Check sheet for the modelled part. Datum: model origin and axes. Units: mm. Face numbers are marked on the shaded views. A direction names the side the tool comes from. Give positions to 0.01 mm unless a question says otherwise; leave off trailing zeros. Order: outer loops, then holes, each group sorted by start corner. A loop starts at its lowest first (then second) coordinate and runs counter-clockwise, first axis right, second up.
Item 1: Sectioned sample at A-A on z = 10. Record the boundary of the cut face in (x, y).
Item 2: Sectioned sample at C-C on y = 26.5. Record the boundary of the cut face in (x, z).
Item 3: Material ranges on line 1 along X through (y, z) = (-8.7, 10); line 2 along X through (y, z) = (16.5, 1.5); line 3 along Z through (x, y) = (5.25, -9.1), recorded low to high.
Item 4: Release check for a two-part mould opening along X. For the marked faces 6, 7 and 8 record: released by +X, released by -X, zero draft, split by the parting line, or undercut.
Item 5: Sectioned sample at B-B on x = -29.75. Record the boundary of the cut face in (y, z), and give its area (3 significant figures).
Item 6: Sectioned sample at D-D on z = 5.75. Record the boundary of the cut face in (x, y).
Item 7: Access from +Z, -Z, +X, -X, +Y, -Y to the whole of each face (thin tool, end or side, straight path). Record for the marked faces 1, 2, 3, 4 and 5.
Item 8: Gauge pin test, flat ends, axial feed: P1, Ø1.8, axis at x = 5.25, z = 10, coming from the +Y side; P2, Ø12, axis at y = 8.5, z = 5.5, coming from the -X side; P3, Ø11.5, axis at x = 5, z = 9.5, coming from the +Y side; P4, Ø5, axis at x = -16, z = 5, coming from the -Y side. Record the tip position at first contact, or that the pin passes through.
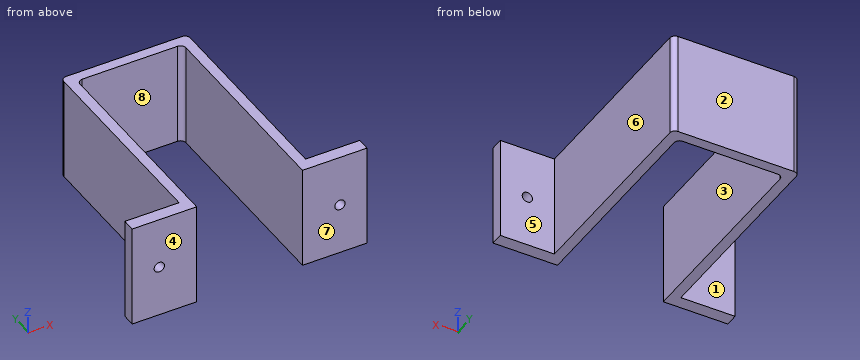
from build123d import *

# Parameters (mm, degrees)
BOSS_EXTRUDE1_DEPTH = 20
FILLET1_R           = 1
SKETCH2_R           = 1
CUT_EXTRUDE1_DEPTH  = 20


with BuildPart() as part:
    # Sketch1 → Boss-Extrude1 (new body)
    with BuildSketch(Plane.XY):
        Polygon((-22.5, -10.265235457), (-22.5, 30.234764543), (-2, 30.234764543), (-2, -10.265235457), (0, -10.265235457), (10.5, -10.265235457), (10.5, -7.797091413), (0, -7.797091413), (0, 32.234764543), (-24.5, 32.234764543), (-24.5, -7.797091413), (-35, -7.797091413), (-35, -10.265235457), (-26.067867036, -10.265235457), align=None)
    extrude(amount=BOSS_EXTRUDE1_DEPTH)

    # Fillet1
    fillet1_edges = [part.edges().sort_by_distance(p)[0] for p in [
        (-22.5, 30.234764543, 10),
        (-2, 30.234764543, 10),
        (0, 32.234764543, 10),
        (-24.5, 32.234764543, 10),
    ]]
    fillet(fillet1_edges, radius=FILLET1_R)

    # Sketch2 → Cut-Extrude1 (cut)
    with BuildSketch(Plane(origin=(0, -7.797091413, 0), x_dir=(1, 0, 0), z_dir=(0, 1, 0))):
        with Locations((-29.75, -10)):
            Circle(SKETCH2_R)
        with Locations((5.25, -10)):
            Circle(SKETCH2_R)
    extrude(amount=-CUT_EXTRUDE1_DEPTH, mode=Mode.SUBTRACT)


solid = part.part
Report:
1. outline: (-35, -10.27) - (-30.75, -10.27) - (-30.75, -7.8) - (-35, -7.8) - close; (-28.75, -10.27) - (-22.5, -10.27) - (-22.5, 29.23) arc R1 cw to (-21.5, 30.23) - (-3, 30.23) arc R1 cw to (-2, 29.23) - (-2, -10.27) - (4.25, -10.27) - (4.25, -7.8) - (0, -7.8) - (0, 31.23) arc R1 ccw to (-1, 32.23) - (-23.5, 32.23) arc R1 ccw to (-24.5, 31.23) - (-24.5, -7.8) - (-28.75, -7.8) - close; (6.25, -10.27) - (10.5, -10.27) - (10.5, -7.8) - (6.25, -7.8) - close
2. outline: (-24.5, 0) - (-22.5, 0) - (-22.5, 20) - (-24.5, 20) - close; (-2, 0) - (0, 0) - (0, 20) - (-2, 20) - close
3. line 1: x = -35 to -30.75, -28.75 to -22.5, -2 to 4.25, 6.25 to 10.5
3. line 2: x = -24.5 to -22.5, -2 to 0
3. line 3: z = 0 to 9, 11 to 20
4. face 6: released by +X
4. face 7: zero draft
4. face 8: undercut
5. outline: (-10.27, 0) - (-7.8, 0) - (-7.8, 9) - (-10.27, 9) - close; (-10.27, 11) - (-7.8, 11) - (-7.8, 20) - (-10.27, 20) - close
5. area: 44.4 mm2
6. outline: (-35, -10.27) - (-22.5, -10.27) - (-22.5, 29.23) arc R1 cw to (-21.5, 30.23) - (-3, 30.23) arc R1 cw to (-2, 29.23) - (-2, -10.27) - (10.5, -10.27) - (10.5, -7.8) - (0, -7.8) - (0, 31.23) arc R1 ccw to (-1, 32.23) - (-23.5, 32.23) arc R1 ccw to (-24.5, 31.23) - (-24.5, -7.8) - (-35, -7.8) - close
7. face 1: +Z, -Z, -X, +Y
7. face 2: +Z, -Z, +X, -X, +Y
7. face 3: +Z, -Z, -Y
7. face 4: +Z, -Z, +X, -X, -Y
7. face 5: +Z, -Z, +X, +Y
8. P1: passes through
8. P2: stops at x = -24.5
8. P3: stops at y = 32.2
8. P4: stops at y = 30.23
